from build123d import *

# Parameters (mm, degrees)
SKETCH1_R           = 1.778
SKETCH1_R_2         = 1.55
SKETCH1_R_3         = 5
BOSS_EXTRUDE1_DEPTH = 6.35
FILLET1_R           = 10


with BuildPart() as part:
    # Sketch1 → Boss-Extrude1 (new body)
    with BuildSketch(Plane.XY):
        with BuildLine():
            Line((75.814774676, 17.433113678), (30, 25))
            Line((30, 25), (0, 25))
            Line((0, 25), (0, 0))
            Line((0, 0), (30, 0))
            Line((30, 0), (75.814763379, 7.566776682))
            ThreePointArc((75.814763379, 7.566776682), (80, 12.499940388), (75.814774676, 17.433113678))
        make_face()
        with Locations((24.779, 12.499946113)):
            Circle(SKETCH1_R, mode=Mode.SUBTRACT)
        with Locations((5.221, 12.499946113)):
            Circle(SKETCH1_R, mode=Mode.SUBTRACT)
        with Locations((75, 12.499946113)):
            Circle(SKETCH1_R_2, mode=Mode.SUBTRACT)
        with Locations((15, 12.499946113)):
            Circle(SKETCH1_R_3, mode=Mode.SUBTRACT)
    extrude(amount=BOSS_EXTRUDE1_DEPTH)

    # Fillet1
    fillet1_edges = [part.edges().sort_by_distance(p)[0] for p in [
        (0, 0, 3.175),
        (0, 25, 3.175),
    ]]
    fillet(fillet1_edges, radius=FILLET1_R)


solid = part.part
Source: CAD feature listing. Evaluate the final solid. Frame: model axes, mm. Give positions to 0.01 mm unless a question says otherwise; leave off trailing zeros. Write each loop counter-clockwise with the first axis right and the second up, starting at its lowest first coordinate (ties: lowest second). Pieces come first, ordered by that corner, then holes. Notation, with made-up numbers: (46, 48) -> (78, 48) arc R17 cw to (78, 53) -> close; hole circle Ø5 at (5.25, 26.25). An arc over 180 degrees is marked (long way). Return JSON: item names as keys, results as strings. Group by question number.
1. Section D-D, the plane y = 23.5. Output: boundary loops of the cut face in (x, z).
2. Pin query (flat end, axial travel): pin 1 Ø1 at (y, z) = (5, 2) entering from -X; pin 2 Ø1.5 at (y, z) = (18.5, 3) entering from -X. Return the tip coordinate at first contact, or that it passes through.
3. Section C-C, the plane y = 8.5. Output: boundary loops of the cut face in (x, z), then the cut area to 3 significant figures.
4. Section B-B, the plane z = 1.5. Output: boundary loops of the cut face in (x, y).
5. Material intervals for line 1 (X direction, y = 13, z = 3.25); line 2 (Y direction, x = 4.5, z = 5.5); line 3 (X direction, y = 8.5, z = 0.5), sorted ascending. Write a range as from..to.
6. Mould query, pull axis X, two halves, no side actions, for faces 1 (the face through (53.228, 21.164, 3.131)), 2 (the face through (20, 0, 3)), 3 (the face through (19.619, 10.585, 3.131)). Classes: +X half, -X half, draft (parallel to the pull), parting line (faces both ways), or undercut.
7. Section A-A, the plane x = 15. Output: boundary loops of the cut face in (y, z).
Determined:
{
 "1": {"outline": "(4.73, 0) -> (39.08, 0) -> (39.08, 6.35) -> (4.73, 6.35) -> close"},
 "2": {"pin 1": "stops at x = 1.07", "pin 2": "stops at x = 0.39"},
 "3": {"outline": "(0.11, 0) -> (12, 0) -> (12, 6.35) -> (0.11, 6.35) -> close; (18, 0) -> (78, 0) -> (78, 6.35) -> (18, 6.35) -> close", "area": "456 mm2"},
 "4": {"outline": "(0, 10) arc R10 ccw to (10, 0) -> (30, 0) -> (75.81, 7.57) arc R5 ccw to (75.81, 17.43) -> (30, 25) -> (10, 25) arc R10 ccw to (0, 15) -> close; hole circle Ø3.56 at (5.22, 12.5); hole circle Ø10 at (15, 12.5); hole circle Ø3.56 at (24.78, 12.5); hole circle Ø3.1 at (75, 12.5)"},
 "5": {"line 1": "x = 0..3.51, 6.93..10.03, 19.97..23.07, 26.49..73.53, 76.47..79.97", "line 2": "y = 1.65..10.87, 14.13..23.35", "line 3": "x = 0.11..12, 18..78"},
 "6": {"face 1": "+X half", "face 2": "draft", "face 3": "undercut"},
 "7": {"outline": "(0, 0) -> (7.5, 0) -> (7.5, 6.35) -> (0, 6.35) -> close; (17.5, 0) -> (25, 0) -> (25, 6.35) -> (17.5, 6.35) -> close"}
}
